Geometry: see drawing. Coordinates: mm, zero at the bounding-box minimum. A direction names the side the tool comes from. Coordinates: 2 decimals unless noted, no trailing zeros. Write each loop counter-clockwise with the first axis right and the second up, starting at its lowest first coordinate (ties: lowest second). Pieces come first, ordered by that corner, then holes. Notation, with made-up numbers: (-5.5, -37.75) -> (48.5, -37.75) arc R26 ccw to (48.5, -4.75) -> close; hole circle Ø6 at (6, 16). An arc over 180 degrees is marked (long way). Answer as a JSON object with one key per item and string values. Group by question number.
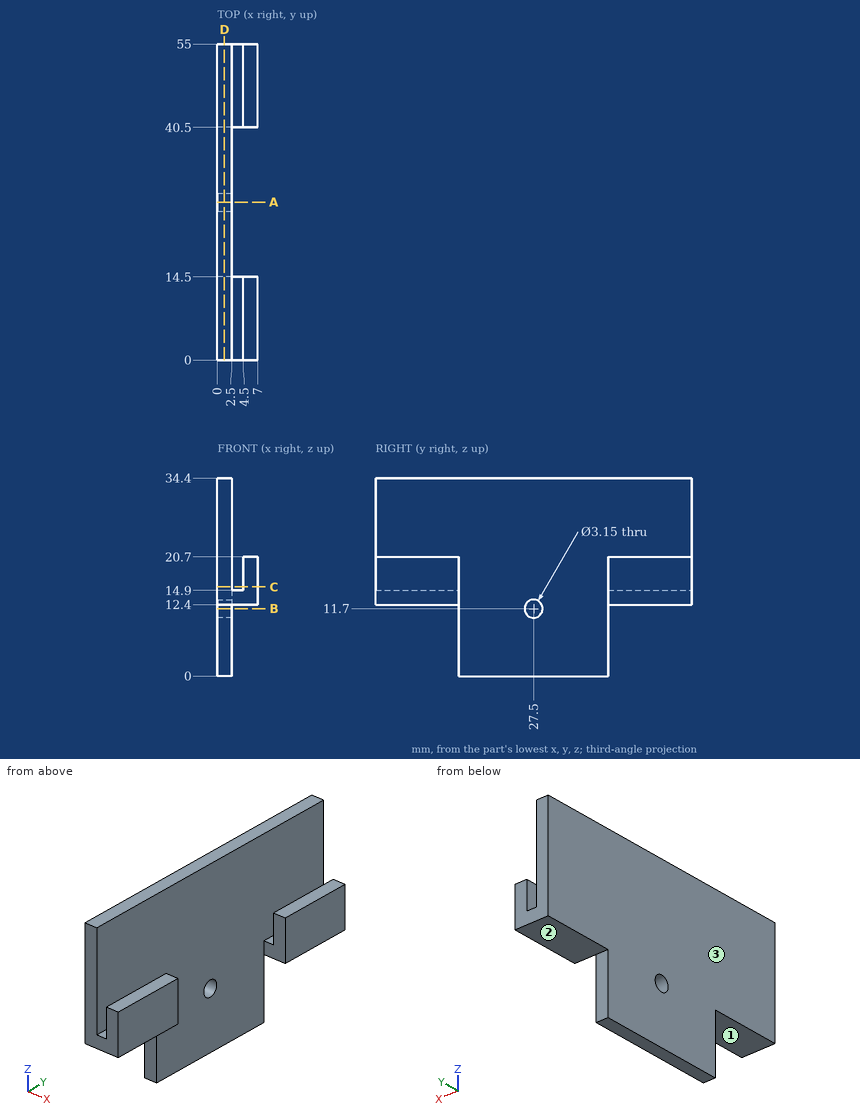
Item 1: Section C-C on z = 15.5. Output: boundary loops of the cut face in (x, y).
Item 2: Section A-A on y = 27.5. Output: boundary loops of the cut face in (x, z) (3 decimals).
Item 3: Section D-D on x = 1.25. Output: boundary loops of the cut face in (y, z) (3 decimals), then the cut area to 3 significant figures.
Item 4: Section B-B on z = 11.7. Output: boundary loops of the cut face in (x, y) (3 decimals), then the cut area to 3 significant figures.
Item 5: Ray query, L1, parallel to Y at x = 1.7, z = 11.7 (3 decimals); L2, parallel to X at y = 49, z = 15; L3, parallel to Z at x = 6.75, y = 9. Return the intervals inside material, ascending. Write a range as [from, to].
Item 6: Contact query for flat-ended pins moving along their axis: pin 1 (10.5 mm diameter, centred on y = 25, z = 16.5, fed in from +X); pin 2 (1.2 mm diameter, centred on x = 2, z = 9.5, fed in from +Y); pin 3 (1.6 mm diameter, centred on x = 3.5, y = 46.5, fed in from +Z). Output: stop coordinate, or through.
Item 7: Set-up query: the marked faces 1, 2 and 3. Return all of +Z, -Z, +X, -X, +Y, -Y with unobstructed straight access to the full face (end or side cutting, diameter ignored); none if empty.
Answer sheet:
{
 "1": {"outline": "(0, 0) -> (2.5, 0) -> (2.5, 55) -> (0, 55) -> close; (4.5, 0) -> (7, 0) -> (7, 14.5) -> (4.5, 14.5) -> close; (4.5, 40.5) -> (7, 40.5) -> (7, 55) -> (4.5, 55) -> close"},
 "2": {"outline": "(0, 0) -> (2.5, 0) -> (2.5, 10.125) -> (0, 10.125) -> close; (0, 13.275) -> (2.5, 13.275) -> (2.5, 34.4) -> (0, 34.4) -> close"},
 "3": {"outline": "(0, 12.4) -> (14.5, 12.4) -> (14.5, 0) -> (40.5, 0) -> (40.5, 12.4) -> (55, 12.4) -> (55, 34.4) -> (0, 34.4) -> close; hole circle Ø3.15 at (27.5, 11.7)", "area": "1,520 mm^2"},
 "4": {"outline": "(0, 14.5) -> (2.5, 14.5) -> (2.5, 25.925) -> (0, 25.925) -> close; (0, 29.075) -> (2.5, 29.075) -> (2.5, 40.5) -> (0, 40.5) -> close", "area": "57.1 mm^2"},
 "5": {"L1": "y = [14.5, 25.925], [29.075, 40.5]", "L2": "x = [0, 2.5], [4.5, 7]", "L3": "z = [12.4, 20.7]"},
 "6": {"pin 1": "stops at x = 2.5", "pin 2": "stops at y = 40.5", "pin 3": "stops at z = 14.9"},
 "7": {"face 1": "-Z, +X, -X, -Y", "face 2": "-Z, +X, -X, +Y", "face 3": "+Z, -Z, -X, +Y, -Y"}
}
